The listing builds one solid part. Answer for the finished solid, in the listing's coordinates (mm). Face numbers are marked on the shaded views. A direction names the side the tool comes from. Coordinates: 2 decimals unless noted, no trailing zeros. Order: outer loops, then holes, each group sorted by start corner. A loop starts at its lowest first (then second) coordinate and runs counter-clockwise, first axis right, second up. Notation, with made-up numbers: (-11.75, 64) -> (42.25, 64) arc R36 cw to (42.25, 99) -> close; hole circle Ø2 at (39.25, 50). An arc over 180 degrees is marked (long way). Answer in a Markdown table with one row per item. Add a question column.
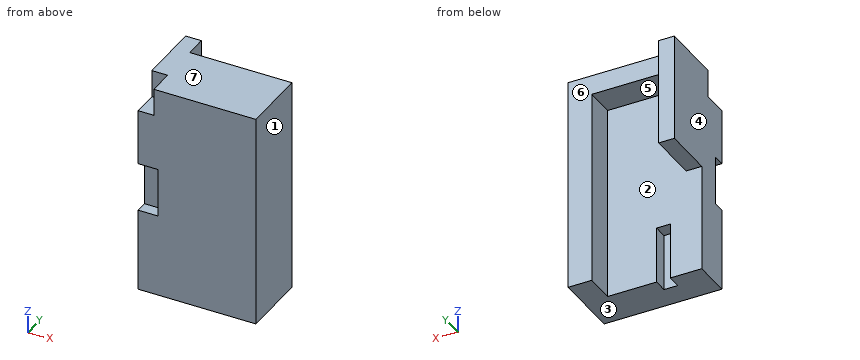
```python
from build123d import *

# Parameters (mm, degrees)
EXTRUDE_1_DEPTH          = 110
SKETCH_2_W               = 8
SKETCH_2_H               = 13
CUT_EXTRUDE_1_DEPTH      = 14
CUT_EXTRUDE_4_DEPTH      = 120.63381629
CUT_EXTRUDE_4_DEPTH_BACK = 15
SKETCH_4_W               = 8
SKETCH_4_H               = 55
SKETCH_5_W               = 7
SKETCH_5_H               = 7
CUT_EXTRUDE_5_DEPTH      = 29
SKETCH_3_W               = 25
SKETCH_3_H               = 6
CUT_EXTRUDE_6_DEPTH      = 10
SKETCH_6_W               = 5
SKETCH_6_H               = 110
CUT_EXTRUDE_7_DEPTH      = 119.30997422


with BuildPart() as part:
    # Эскиз1 → Бобышка-Вытянуть1 (new body)
    with BuildSketch(Plane.XY):
        Polygon((-32.5, 22.5), (-32.5, -22.5), (32.5, -22.5), (32.5, -6.5), (27.5, -6.5), (27.5, 11.5), (-24.5, 11.5), (-24.5, 22.5), align=None)
    extrude(amount=EXTRUDE_1_DEPTH)

    # Эскиз2 → Вырез-Вытянуть1 (cut)
    with BuildSketch(Plane.XY.offset(110)):
        with Locations((-28.5, -16)):
            Rectangle(SKETCH_2_W, SKETCH_2_H)
    extrude(amount=-CUT_EXTRUDE_1_DEPTH, mode=Mode.SUBTRACT)

    # Эскиз4 → Вырез-Вытянуть4 (cut, two sides: drawn at the far end of the back side and taken through both)
    with BuildSketch(Plane(origin=(0, 11.5, 0), x_dir=(1, 0, 0), z_dir=(0, 1, 0)).offset(-CUT_EXTRUDE_4_DEPTH_BACK)):
        Polygon((-24.5, -55), (-24.5, -100), (15.5, -100), (15.5, 0), (-24.5, 0), align=None)
        with Locations((-28.5, -27.5)):
            Rectangle(SKETCH_4_W, SKETCH_4_H)
    extrude(amount=CUT_EXTRUDE_4_DEPTH + CUT_EXTRUDE_4_DEPTH_BACK, mode=Mode.SUBTRACT)

    # Эскиз5 → Вырез-Вытянуть5 (cut)
    with BuildSketch(Plane(origin=(0, 0, 0), x_dir=(-1, 0, 0), z_dir=(0, 0, -1))):
        with Locations((13, -7)):
            Rectangle(SKETCH_5_W, SKETCH_5_H)
    extrude(amount=-CUT_EXTRUDE_5_DEPTH, mode=Mode.SUBTRACT)

    # Эскиз3 → Вырез-Вытянуть6 (cut)
    with BuildSketch(Plane(origin=(-32.5, 0, 0), x_dir=(0, 0, -1), z_dir=(1, 0, 0))):
        with Locations((-55, -19.5)):
            Rectangle(SKETCH_3_W, SKETCH_3_H)
    extrude(amount=CUT_EXTRUDE_6_DEPTH, mode=Mode.SUBTRACT)

    # Эскиз6 → Вырез-Вытянуть7 (cut, through all)
    with BuildSketch(Plane(origin=(0, -6.5, 0), x_dir=(1, 0, 0), z_dir=(0, 1, 0))):
        with Locations((30, -55)):
            Rectangle(SKETCH_6_W, SKETCH_6_H)
    extrude(amount=-CUT_EXTRUDE_7_DEPTH, mode=Mode.SUBTRACT)


solid = part.part
```
Q1. Straight lines are drawn through the part: line 1 (X direction, y = -1, z = 78.5); line 2 (Y direction, x = 16, z = 55.5); line 3 (Y direction, x = 9, z = 14). For each, find the intervals that lie inside material, in ascending order.
Q2. Determine the mould class of the marked faces 1, 2, 3 and 4 for opening direction X: +X half, -X half, draft (parallel to the pull), parting line (faces both ways), or undercut.
Q3. For the marked faces 5, 6 and 7, determine the directions among +Z, -Z, +X, -X, +Y, -Y from which every point of the face is accessible in a straight line to the end or side of a thin tool.
Q4. A cutting plane is placed at C-C (z = 9). Determine the outline of the cut face in (x, y).
Q5. A cutting plane is placed at A-A (y = -6.5). Determine the outline of the cut face in (x, z).
Q6. A cutting plane is placed at B-B (x = -11.5). Determine the outline of the cut face in (y, z).
Q7. A cutting plane is placed at D-D (x = 8). Determine the outline of the cut face in (y, z).
Q8. Given pin 1 (2.5 mm diameter, centred on x = -30.5, y = 8, fed in from -Z); pin 2 (7.5 mm diameter, centred on y = 7, z = 30, fed in from -X); pin 3 (11 mm diameter, centred on x = -29, z = 59, fed in from -Y), each flat-ended and moving along its own axis, determine where each tip first touches the part or whether it passes through.
Returned:
| question | item | result |
|---|---|---|
| 1 | line 1 | x = -32.5 to -24.5, 15.5 to 27.5 |
| 1 | line 2 | y = -22.5 to 11.5 |
| 1 | line 3 | y = -22.5 to -3.5 |
| 2 | face 1 | +X half |
| 2 | face 2 | undercut |
| 2 | face 3 | draft |
| 2 | face 4 | -X half |
| 3 | face 5 | -Z, +Y |
| 3 | face 6 | +Z, -Z, +X, +Y |
| 3 | face 7 | +Z, +X, -X, +Y, -Y |
| 4 | outline | (-32.5, -22.5) -> (27.5, -22.5) -> (27.5, 11.5) -> (15.5, 11.5) -> (15.5, -3.5) -> (-9.5, -3.5) -> (-9.5, -10.5) -> (-16.5, -10.5) -> (-16.5, -3.5) -> (-32.5, -3.5) -> close |
| 5 | outline | (-32.5, 0) -> (-16.5, 0) -> (-16.5, 29) -> (-9.5, 29) -> (-9.5, 0) -> (27.5, 0) -> (27.5, 110) -> (-32.5, 110) -> close |
| 6 | outline | (-22.5, 0) -> (-10.5, 0) -> (-10.5, 29) -> (-3.5, 29) -> (-3.5, 100) -> (11.5, 100) -> (11.5, 110) -> (-22.5, 110) -> close |
| 7 | outline | (-22.5, 0) -> (-3.5, 0) -> (-3.5, 100) -> (11.5, 100) -> (11.5, 110) -> (-22.5, 110) -> close |
| 8 | pin 1 | stops at z = 55 |
| 8 | pin 2 | stops at x = 15.5 |
| 8 | pin 3 | stops at y = -16.5 |
